Work out the finished part from the listing and answer in its coordinate system (mm). A direction names the side the tool comes from. Coordinates: 2 decimals unless noted, no trailing zeros. Loops run counter-clockwise (first coordinate to the right, second up) from the corner with the lowest first, then second, coordinate; pieces in that order, holes last. Notation, with made-up numbers: (83.5, -13) -> (112.5, -13) arc R19 cw to (112.5, 9) -> close; hole circle Ø4 at (82.25, 76). An arc over 180 degrees is marked (long way). Use a Markdown table: item, result.
Autodesk Inventor part; units mm, degrees
ref_plane "YZ Plane" through (0, 0, 0) normal (1, 0, 0) x (0, 1, 0)
ref_plane "XZ Plane" through (0, 0, 0) normal (0, 1, 0) x (-1, 0, 0)
ref_plane "XY Plane" through (0, 0, 0) normal (0, 0, 1) x (1, 0, 0)
sketch "Sketch5" plane through (0, 0, 0) normal (0, 0, 1) x (1, 0, 0)
  line L0 (0, 0) -> (8.255, 0)
  circle A0 centre (8.255, 0) radius 1.27
  circle A1 centre (0, -8.255) radius 1.27
  circle A2 centre (-8.255, 0) radius 1.27
  line L1 (0, 0) -> (-23.6329, 0)
  line L2 (-23.6329, 0) -> (-15.3779, 0)
  circle A3 centre (-15.3779, 0) radius 1.27
  circle A4 centre (-23.6329, -8.255) radius 1.27
  circle A5 centre (-31.8879, 0) radius 1.27
  circle A6 centre (-31.8879, 0) radius 3.4925
  circle A7 centre (-23.6329, -8.255) radius 3.4925
  circle A8 centre (-15.3779, 0) radius 3.4925
  circle A9 centre (-8.255, 0) radius 3.4925
  circle A10 centre (0, -8.255) radius 3.4925
  circle A11 centre (8.255, 0) radius 3.4925
  circle A12 centre (-23.6329, 0) radius 4.7625
  circle A13 centre (0, 0) radius 4.7625
  line L3 (-32.4252, 3.4509) -> (-24.3656, 4.7058)
  line L4 (-22.9002, 4.7058) -> (-14.8406, 3.4509)
  line L5 (-8.7923, 3.4509) -> (-0.7327, 4.7058)
  line L6 (0.7327, 4.7058) -> (8.7923, 3.4509)
  arc A14 (8.7788, -3.453) -> (3.453, -8.7788) centre (9.7312, -9.7312) ccw
  arc A15 (-3.453, -8.7788) -> (-8.7788, -3.453) centre (-9.7312, -9.7312) ccw
  arc A16 (-14.8541, -3.453) -> (-20.1799, -8.7788) centre (-13.9017, -9.7312) ccw
  arc A17 (-27.0859, -8.7788) -> (-32.4117, -3.453) centre (-33.3641, -9.7312) ccw
  line L7 (-14.8406, 3.4509) -> (-8.7923, 3.4509)
  line L8 (-14.8541, -3.453) -> (-8.7788, -3.453)
  dimension "d45" = 8.255
  dimension "d46" = 2.54
  dimension "d49" = 180
  dimension "d51" = 23.6329
  dimension "d52" = 8.255
  dimension "d53" = 2.54
  dimension "d56" = 180
  dimension "d58" = 6.985
  dimension "d59" = 6.985
  dimension "d60" = 6.985
  dimension "d61" = 6.985
  dimension "d62" = 6.985
  dimension "d63" = 6.985
  dimension "d64" = 9.525
  dimension "d65" = 9.525
  dimension "d66" = 6.35
  dimension "d67" = 6.35
  dimension "d68" = 6.35
  dimension "d69" = 6.35
extrude "Extrusion7" add sketch "Sketch5" along normal blind 6.985 contours L1 A13 L0 | L0 A13 L1 | A13 L6 A11 | A11 | A11 A14 A10 A13 | A9 L1 A2 | L1 A2 A9 | A13 A10 A15 A9 | A9 L5 A13 | A10 | A9 L1 A8 L7 | L8 A8 L1 A9 | A8 L1 A3 | A8 A12 L4 | A16 A7 A12 A8 | A8 L1 A3 | A12 | A7 | A7 A17 A6 A12 | A12 A6 L3 | A6
sketch "Sketch6" plane through (0, 0, 6.985) normal (0, 0, 1) x (1, 0, 0)
  circle A0 centre (0, 0) radius 1.8415
  circle A1 centre (0, 0) radius 3.3655
  circle A2 centre (-23.6329, 0) radius 1.8415
  circle A3 centre (-23.6329, 0) radius 3.3655
  dimension "d72" = 3.683
  dimension "d73" = 6.731
  dimension "d74" = 23.6329
  dimension "d75" = 3.683
  dimension "d76" = 6.731
extrude "Extrusion8" cut sketch "Sketch6" against normal through all contours A0 | A2
extrude "Extrusion9" cut sketch "Sketch6" against normal blind 3.175
equation "\"d59\" = d58"
equation "\"d60\" = d58"
equation "\"d61\" = d58"
equation "\"d62\" = d58"
equation "\"d63\" = d58"
equation "\"d67\" = d66"
equation "\"d68\" = d66"
equation "\"d69\" = d66"
properties part number "carriageIdlerPinionExtension" material "ABS Plastic"
Q1. Section B-B on z = 2.25 is taken. State how many separate pieces and enclosed holes the cut face has, and give its area (3 significant figures).
Solved:
| item | result |
|---|---|
| separate pieces | 1 |
| enclosed holes | 8 |
| area | 424 mm² |
Q2. Consider line 1 (Y direction, x = 1, z = 6); line 2 (X direction, y = -8, z = 5.25); line 3 (X direction, y = 2.75, z = 6). Determine where each line is inside the solid, lowest interval first. Write a range as [from, to].
Solved:
| item | result |
|---|---|
| line 1 | [-11.6, -9.04], [-7.47, -3.21], [3.21, 4.66] |
| line 2 | [-27.25, -24.88], [-22.39, -20.01], [-3.62, -1.24], [1.24, 3.62] |
| line 3 | [-34.04, -25.57], [-21.69, -1.94], [1.94, 10.41] |
Q3. Section D-D on y = -5.5 is taken. Determine the outline of the cut face in (x, z) (3 decimals), and give its area (3 significant figures).
Solved:
| item | result |
|---|---|
| outline | (-28.629, 0) -> (-18.637, 0) -> (-18.637, 6.985) -> (-28.629, 6.985) -> close; (-4.996, 0) -> (4.996, 0) -> (4.996, 6.985) -> (-4.996, 6.985) -> close |
| area | 140 mm² |
Q4. For faces 5 (the flat face through (-12, 3.451, 3)), 6 (the flat face through (4.706, 4.087, 3.444)), 7 (the flat face through (-22.2, -1.4, 3.81)), 8 (the cylindrical face through (0.85, -1.634, 1.932)), 9 (the flat face through (-12, -3.453, 3)), determine the directions among +Z, -Z, +X, -X, +Y, -Y from which every point of the face is accessible in a straight line to the end or side of a thin tool.
Solved:
| item | result |
|---|---|
| face 5 | +Z, -Z, +Y |
| face 6 | +Z, -Z, +X, +Y |
| face 7 | +Z |
| face 8 | +Z, -Z |
| face 9 | +Z, -Z, -Y |
Q5. Given pin 1 Ø2 at (x, y) = (-1, 0) entering from +Z; pin 2 Ø1.8 at (x, z) = (-11, 3.5) entering from -Y, each flat-ended and moving along its own axis, determine where each tip first touches the part or whether it passes through.
Solved:
| item | result |
|---|---|
| pin 1 | z = 3.81 |
| pin 2 | y = -3.45 |
Q6. Section A-A on x = 0 is taken. Determine the outline of the cut face in (y, z) (1 decimal).
Solved:
| item | result |
|---|---|
| outline | (-11.7, 0) -> (-9.5, 0) -> (-9.5, 7) -> (-11.7, 7) -> close; (-7, 0) -> (-1.8, 0) -> (-1.8, 3.8) -> (-3.4, 3.8) -> (-3.4, 7) -> (-7, 7) -> close; (1.8, 0) -> (4.8, 0) -> (4.8, 7) -> (3.4, 7) -> (3.4, 3.8) -> (1.8, 3.8) -> close |
Q7. Determine the mould class of faces 1 (the flat face through (-12, -2, 6.985)), 2 (the cylindrical face through (-23.643, 4.762, 3.444)), 3 (the cylindrical face through (-35.38, -0.08, 3.44)), 4 (the cylindrical face through (11.747, 0.063, 3.444)) for opening direction X: pulls with the +X half, pulls with the -X half, needs draft (parallel to the pull), parting line crosses it, or undercut.
Solved:
| item | result |
|---|---|
| face 1 | needs draft |
| face 2 | undercut |
| face 3 | pulls with the -X half |
| face 4 | pulls with the +X half |
